Can you work these out from the model? Positions are in its coordinate system, mm. A direction names the side the tool comes from. Round coordinates to 2 decimals unless told otherwise and drop trailing zeros. Write each loop counter-clockwise with the first axis right and the second up, starting at its lowest first coordinate (ties: lowest second). Pieces come first, ordered by that corner, then holes. Notation, with made-up numbers: M 76.5,42.25 L 94.5,42.25 A31 ccw 94.5,69.25 Z; hole C 78,57.25 d3. An arc over 180 degrees is marked long. Answer in a Markdown table with one row per item. Add a question column.
(1) I'm going to push flat-ended pins straight in: pin 1 (1 mm diameter, centred on y = -1, z = -10, fed in from +X); pin 2 (1 mm diameter, centred on y = -2, z = 1.5, fed in from +X); pin 3 (1 mm diameter, centred on y = -1, z = 3.5, fed in from +X). Where does each tip first touch, or does it pass through?
(2) Suppose I cut it at A-A, the plane x = 19.05. Write out the boundary of the cut face in (y, z) (3 decimals).
(3) If we mould it in two halves opening along X, with no side actions, what happens to faces 1 (the face through (26.67, -1.57, -3.96)), 2 (the face through (-4, -3.175, -4)), 3 (the face through (20.32, -2, -10))? For each: released by +X, released by -X, zero draft, split by the parting line, or undercut.
(4) Suppose I cut it at B-B, the plane y = -2.15. Write out the boundary of the cut face in (x, z) (3 decimals).
(5) If I drill on probe 1 along Z at (x, y) = (19.05, -1.25) (3 decimals); probe 2 along X at (y, z) = (-1.4, -2.25); probe 3 along X at (y, z) = (-1.5, -6.25), over which ranges is the centre line in solid material (lowest first)?
(6) For faces 4 (the face through (-4, 0, -4)), 5 (the face through (20.32, -2, 3)), 6 (the face through (19, -2, -9.525)), which set-ups out of +Z, -Z, +X, -X, +Y, -Y let a thin tool reach every point of the face, with its end or its side?
(7) Suppose I cut it at C-C, the plane z = -3.81. Write out the boundary of the cut face in (x, y) (3 decimals), then the cut area to 3 significant figures.
from build123d import *

# Parameters (mm, degrees)
F0_R     = 1.778
F1_DEPTH = 3.175


with BuildPart() as f1:
    # F0 (on Front) → F1 (new body)
    with BuildSketch(Plane.XZ):
        with BuildLine():
            Line((17.78, 1.905), (17.78, 3.81))
            Line((17.78, 3.81), (-33.02, 3.81))
            Line((-33.02, 3.81), (-33.02, -11.43))
            Line((-33.02, -11.43), (17.78, -11.43))
            Line((17.78, -11.43), (17.78, -9.525))
            Line((17.78, -9.525), (20.32, -9.525))
            Line((20.32, -9.525), (20.32, -11.323421))
            ThreePointArc((20.32, -11.323421), (26.67, -3.81), (20.32, 3.703421))
            Line((20.32, 3.703421), (20.32, 1.905))
            Line((20.32, 1.905), (17.78, 1.905))
        make_face()
        with Locations((19.05, -3.81)):
            Circle(F0_R, mode=Mode.SUBTRACT)
    extrude(amount=F1_DEPTH)


solid = f1.part
Calculated:
| question | item | result |
|---|---|---|
| 1 | pin 1 | x = 24.12 |
| 1 | pin 2 | x = 24.96 |
| 1 | pin 3 | x = 22.47 |
| 2 | outline | M -3.175,-9.525 L 0,-9.525 L 0,-5.588 L -3.175,-5.588 Z; M -3.175,-2.032 L 0,-2.032 L 0,1.905 L -3.175,1.905 Z |
| 3 | face 1 | released by +X |
| 3 | face 2 | zero draft |
| 3 | face 3 | undercut |
| 4 | outline | M -33.02,-11.43 L 17.78,-11.43 L 17.78,-9.525 L 20.32,-9.525 L 20.32,-11.323 A7.62 ccw 20.32,3.703 L 20.32,1.905 L 17.78,1.905 L 17.78,3.81 L -33.02,3.81 Z; hole C 19.05,-3.81 d3.556 |
| 5 | probe 1 | -9.525 to -5.588, -2.032 to 1.905 |
| 5 | probe 2 | -33.02 to 18.2, 19.9 to 26.51 |
| 5 | probe 3 | -33.02 to 26.27 |
| 6 | face 4 | +Z, -Z, +X, -X, +Y |
| 6 | face 5 | +Z, +Y, -Y |
| 6 | face 6 | -Z, +Y, -Y |
| 7 | outline | M -33.02,-3.175 L 17.272,-3.175 L 17.272,0 L -33.02,0 Z; M 20.828,-3.175 L 26.67,-3.175 L 26.67,0 L 20.828,0 Z |
| 7 | area | 178 mm² |
